```python
from build123d import *

# Parameters (mm, degrees)
SKETCH1_R               = 38.1
BOSS_EXTRUDE1_DEPTH     = 12.7
SKETCH2_W               = 2.54
SKETCH2_H               = 46.36082965
CUT_EXTRUDE_THIN2_DEPTH = 2.54


with BuildPart() as part:
    # Sketch1 → Boss-Extrude1 (new body)
    with BuildSketch(Plane(origin=(0, 0, 0), x_dir=(1, 0, 0), z_dir=(0, 1, 0))):
        Circle(SKETCH1_R)
    extrude(amount=BOSS_EXTRUDE1_DEPTH)

    # Sketch2 → Cut-Extrude-Thin2 (cut)
    with BuildSketch(Plane(origin=(0, 12.7, 0), x_dir=(1, 0, 0), z_dir=(0, 1, 0))):
        with Locations((0, 23.180414825)):
            Rectangle(SKETCH2_W, SKETCH2_H)
    extrude(amount=-CUT_EXTRUDE_THIN2_DEPTH, mode=Mode.SUBTRACT)


solid = part.part
```
Input: part model. Units: mm. Frame: model coordinates. A direction names the side the tool comes from. Coordinates: 2 decimals unless noted, no trailing zeros. Loops run counter-clockwise (first coordinate to the right, second up) from the corner with the lowest first, then second, coordinate; pieces in that order, holes last. Notation, with made-up numbers: M 48.5,56.25 L 107.5,56.25 A30 ccw 107.5,79.25 Z; hole C 24,33 d4. An arc over 180 degrees is marked long. One line per item, written item: value.
(1) Pin query (flat end, axial travel): pin 1 (0.8 mm diameter, centred on y = 11.5, z = -11.5, fed in from +X); pin 2 (1.3 mm diameter, centred on x = 0, z = -18, fed in from +Y); pin 3 (2 mm diameter, centred on x = -27.5, y = 8.5, fed in from +Z). Return the tip coordinate at first contact, or that it passes through.
Filled in:
pin 1: x = 36.45
pin 2: y = 10.16
pin 3: z = 27.37
(2) Pull-direction query (X, two-part tool) for faces 1 (the flat face through (0, 10.16, -19)), 2 (the flat face through (1.27, 11, -19)), 3 (the flat face through (-1, 0, -1)), 4 (the cylindrical face through (-30.235, 6.261, 23.183)); classes: +X half, -X half, draft (parallel to the pull), parting line (faces both ways), or undercut.
Filled in:
face 1: undercut
face 2: undercut
face 3: draft
face 4: parting line
(3) Section C-C (y = 1.75). Output: boundary loops of the cut face in (x, z).
Filled in:
outline: C 0,0 d76.2
(4) Section A-A (x = 0). Output: boundary loops of the cut face in (y, z).
Filled in:
outline: M 0,-38.1 L 10.16,-38.1 L 10.16,0 L 12.7,0 L 12.7,38.1 L 0,38.1 Z
(5) Line query: line 1 along X through (y, z) = (11.75, -10); line 2 along X through (y, z) = (3.5, 29); line 3 along X through (y, z) = (4.75, 30). Output: solid intervals per line, ascending. Write a range as from..to.
Filled in:
line 1: -36.76..-1.27, 1.27..36.76
line 2: -24.71..24.71
line 3: -23.49..23.49
(6) Section B-B (z = -7.5). Output: boundary loops of the cut face in (x, y), and give its area (3 significant figures).
Filled in:
outline: M -37.35,0 L 37.35,0 L 37.35,12.7 L 1.27,12.7 L 1.27,10.16 L -1.27,10.16 L -1.27,12.7 L -37.35,12.7 Z
area: 942 mm^2
(7) Reachability of faces 5 (the flat face through (0, 11, 0)), 6 (the flat face through (-1, 12.7, 8)) from +Z, -Z, +X, -X, +Y, -Y: full face, straight path, thin tool, end or side. Return the list, or none.
Filled in:
face 5: -Z, +Y
face 6: +Z, -Z, +X, -X, +Y
(8) Section D-D (x = -24). Output: boundary loops of the cut face in (y, z), and give its area (3 significant figures).
Filled in:
outline: M 0,-29.59 L 12.7,-29.59 L 12.7,29.59 L 0,29.59 Z
area: 752 mm^2
